Here's how the part is built. I have some questions about the finished solid (model axes, mm). A direction names the side the tool comes from. Round coordinates to 2 decimals unless told otherwise and drop trailing zeros. Write each loop counter-clockwise with the first axis right and the second up, starting at its lowest first coordinate (ties: lowest second). Pieces come first, ordered by that corner, then holes. Notation, with made-up numbers: (-29.5, 58.25) -> (-25.5, 58.25) arc R22 ccw to (-25.5, 77.25) -> close; hole circle Ø8 at (-5, 64). An arc over 180 degrees is marked (long way). Put each result on its own line as item: value. Start each with the question number.
1) I want a section at B-B, the plane z = 17.25. List the corners of the cut face in (x, y) for me.
2) I want a section at A-A, the plane y = -57.5. List the corners of the cut face in (x, z) for me.
3) Which directions (+Z, -Z, +X, -X, +Y, -Y) give clear straight access to the entire face, cutting with the end or side of a thin tool? Please do faces 5 (the flat face through (0.1, -81.3, -4)), 6 (the flat face through (-13, 37, 0)), 7 (the cylindrical face through (-1.421, 38.974, 7.395)).
4) Will these pins go through, and if not, where does the flat tip stop? P1, Ø5, axis at x = -4.5, z = -1, coming from the +Y side; P2, Ø3, axis at y = -62.5, z = 17.5, coming from the -X side; P3, Ø3, axis at y = -27, z = 7, coming from the +X side.
5) I want a section at C-C, the plane x = 0. List the corners of the cut face in (y, z) for me.
6) We'd pull the mould along X, two halves only. Please class faces 1 (the flat face through (0, -86, 8)), 2 (the flat face through (1, -20, 15)), 3 (the flat face through (-25, -61, 8)), 4 (the flat face through (25, -61, 8)): released by +X, released by -X, zero draft, split by the parting line, or undercut.
7) If I drill on line 1 along X through (y, z) = (0, 3.25); line 2 along X through (y, z) = (-40.5, 6); line 3 along Z through (x, y) = (1.5, -69), over which ranges is the centre line in solid material (lowest first)? Write a range as [from, to].
from build123d import *

# Parameters (mm, degrees)
BOSS_EXTRUDE1_DEPTH = 20
CUT_EXTRUDE1_DEPTH  = 15
BOSS_EXTRUDE2_DEPTH = 4


with BuildPart() as part:
    # Sketch2 → Boss-Extrude1 (new body)
    with BuildSketch(Plane.XY):
        with BuildLine():
            ThreePointArc((44, 0), (-20.4450483, 38.961519478), (-25, -36.20773398))
            ThreePointArc((-25, -36.20773398), (0, -44), (25, -36.20773398))
            ThreePointArc((25, -36.20773398), (38.961519478, -20.4450483), (44, 0))
        make_face()
        with BuildLine():
            ThreePointArc((-25, -36.20773398), (0, -44), (25, -36.20773398))
            Line((25, -36.20773398), (25, -86))
            Line((25, -86), (-25, -86))
            Line((-25, -86), (-25, -36.20773398))
        make_face()
    extrude(amount=BOSS_EXTRUDE1_DEPTH)

    # Sketch3 → Cut-Extrude1 (cut)
    with BuildSketch(Plane(origin=(0, 0, 0), x_dir=(-1, 0, 0), z_dir=(0, 0, -1))):
        with BuildLine():
            Line((-20, -33.481338086), (-20, -81))
            Line((-20, -81), (20, -81))
            Line((20, -81), (20, -33.481338086))
            ThreePointArc((20, -33.481338086), (0, 39), (-20, -33.481338086))
        make_face()
    extrude(amount=-CUT_EXTRUDE1_DEPTH, mode=Mode.SUBTRACT)

    # Sketch4 → Boss-Extrude2 (add)
    with BuildSketch(Plane(origin=(0, 0, 0), x_dir=(-1, 0, 0), z_dir=(0, 0, -1))):
        Polygon((-20, -36.20773398), (-25, -36.20773398), (-25, -86), (25, -86), (25, -36.20773398), (20, -36.20773398), (20, -81), (-20, -81), align=None)
    extrude(amount=BOSS_EXTRUDE2_DEPTH)


solid = part.part
Findings:
1. outline: (-25, -86) -> (25, -86) -> (25, -36.21) arc R44 ccw (long way) to (-25, -36.21) -> close
2. outline: (-25, -4) -> (-20, -4) -> (-20, 15) -> (20, 15) -> (20, -4) -> (25, -4) -> (25, 20) -> (-25, 20) -> close
3. face 5: -Z, +X, -X, +Y, -Y
3. face 6: -Z, +X, -X, +Y
3. face 7: -Z
4. P1: stops at y = 43.94
4. P2: stops at x = -25
4. P3: stops at x = 35.86
5. outline: (-86, -4) -> (-81, -4) -> (-81, 15) -> (39, 15) -> (39, 0) -> (44, 0) -> (44, 20) -> (-86, 20) -> close
6. face 1: zero draft
6. face 2: undercut
6. face 3: released by -X
6. face 4: released by +X
7. line 1: x = [-44, -39], [39, 44]
7. line 2: x = [-25, -20], [20, 25]
7. line 3: z = [15, 20]
